from build123d import *

# Parameters (mm, degrees)
F1_DEPTH      = 125.4125
F2_T          = -15.875
F4_DEPTH      = 125.4125
F5_T          = -15.875
F7_W          = 60.6690326877
F7_H          = 3.0675412395
F8_DEPTH      = 182.626
F8_DEPTH_BACK = 25.4


# Not quite as in the source:
# - a shell that OpenCascade refuses in one call is made with other operations: the cavity is built on its own and cut out


with BuildPart() as f1:
    # F0 (on Top) → F1 (new body)
    with BuildSketch(Plane.XY):
        Polygon((41.9354, 38.1), (-41.9354, 38.1), (-41.9354, -38.1), align=None)
        Polygon((41.9354, -38.1), (41.9354, 38.1), (-41.9354, -38.1), align=None)
    extrude(amount=F1_DEPTH)

    # F2
    f2_openings = [f1.faces().sort_by_distance(p)[0] for p in [
        (0, 0, 125.4125),
    ]]
    offset(amount=F2_T, openings=f2_openings)

    # F3 (on Top) → F4 (join)
    with BuildSketch(Plane.XY):
        Polygon((42.0021460263, -98.425), (-41.8686539737, -38.1), (-41.8686539737, -98.425), align=None)
        Polygon((42.0021460263, -38.1), (-41.8686539737, -38.1), (42.0021460263, -98.425), align=None)
    extrude(amount=F4_DEPTH)

    # F5: a shell. OpenCascade refuses it in one call, so the cavity is built on its own and cut out:
    # the body offset inwards by the wall thickness, plus a prism from it out through each open face.
    f5_core = offset(f1.part, amount=F5_T, kind=Kind.INTERSECTION, mode=Mode.PRIVATE)
    f5_exits = [f5_core.faces().sort_by_distance(p)[0] for p in [
        (0.054837, -60.331537, 109.5375),
    ]]
    add(f5_core, mode=Mode.SUBTRACT)
    extrude(f5_exits, amount=-F5_T, mode=Mode.SUBTRACT)

    # F7 (on offset) → F8 (cut, two sides)
    with BuildSketch(Plane.XZ.offset(123.825)) as f8_sk:
        with Locations((0.2376296824, 119.1418357193)):
            Rectangle(F7_W, F7_H)
    extrude(amount=-F8_DEPTH, mode=Mode.SUBTRACT)
    extrude(f8_sk.sketch, amount=F8_DEPTH_BACK, mode=Mode.SUBTRACT)


solid = f1.part
Model file for the job. Use its own axes, mm. A direction names the side the tool comes from. Coordinates: 2 decimals unless noted, no trailing zeros. Write each loop counter-clockwise with the first axis right and the second up, starting at its lowest first coordinate (ties: lowest second). Pieces come first, ordered by that corner, then holes. Notation, with made-up numbers: (-19, 60.5) - (1, 60.5) arc R30 ccw to (1, 94.5) - close; hole circle Ø1 at (12, 57). An arc over 180 degrees is marked (long way). Write each question's results on one line, items separated by ' | '. Start each with the question number.
1) Flat gauge pins, fed straight in: P1, Ø18, axis at y = -63.5, z = 92, coming from the -X side; P2, Ø12, axis at x = 7.5, y = -49.5, coming from the +Z side (3 decimals); P3, Ø23, axis at y = 9.5, z = 54.5, coming from the +X side. Where does each tip first touch, or does it go through?
2) Cut at A-A (x = -23). Count the separate pieces of the cut face and the enclosed holes in it, then the cut area to 3 significant figures.
3) 3-axis set-ups, long thin cutter, end or side, ignore diameter. For faces 1 (the face through (-1, -29, 125.412)), 2 (the face through (-25.994, -60, 123)): which of +Z, -Z, +X, -X, +Y, -Y reach the whole face in a straight line?
4) Probe line 1 along Y through (x, z) = (-25.5, 57.5) (3 decimals); line 2 along X through (y, z) = (-64.5, 83); line 3 along Z through (x, y) = (-24.5, -90). List the from-to ranges inside material, lowest first. Write a range as from..to.
5) Mould opens along X. For faces 3 (the face through (-1, -29, 0)), 4 (the face through (0, -38.1, 123)), 5 (the face through (42.002, -69, 62)) say: pulls with the +X half, pulls with the -X half, needs draft (parallel to the pull), parting line crosses it, or undercut.
6) Cut at D-D (z = 35.5). Write the cut outline in (x, y) (3 decimals).
7) Cut at B-B (y = -89). Write the cut outline in (x, z).
8) Cut at C-C (x = 28). Write the cut outline in (y, z) (1 decimal).
Returned:
1) P1: x = -41.87 | P2: z = 15.875 | P3: x = 41.94
2) separate pieces: 4 | enclosed holes: 0 | area: 7,240 mm^2
3) face 1: +Z, +X, -X, +Y, -Y | face 2: +Z
4) line 1: -98.425..-82.55, -38.1..-22.225, 22.225..38.1 | line 2: -41.87..-25.99, 26.13..42 | line 3: 0..117.61, 120.68..125.41
5) face 3: needs draft | face 4: undercut | face 5: pulls with the +X half
6) outline: (-41.935, -38.1) - (-41.869, -38.1) - (-41.869, -98.425) - (42.002, -98.425) - (42.002, -38.1) - (41.935, -38.1) - (41.935, 38.1) - (-41.935, 38.1) - close; hole (-26.06, -22.225) - (26.06, -22.225) - (26.06, 22.225) - (-26.06, 22.225) - close; hole (-25.994, -82.55) - (26.127, -82.55) - (26.127, -53.975) - (26.06, -53.975) - (26.06, -38.1) - (-25.994, -38.1) - close
7) outline: (-41.87, 0) - (42, 0) - (42, 125.41) - (-41.87, 125.41) - close; hole (-30.1, 117.61) - (30.57, 117.61) - (30.57, 120.68) - (-30.1, 120.68) - close
8) outline: (-98.4, 0) - (38.1, 0) - (38.1, 117.6) - (-98.4, 117.6) - close; (-98.4, 120.7) - (38.1, 120.7) - (38.1, 125.4) - (-98.4, 125.4) - close
